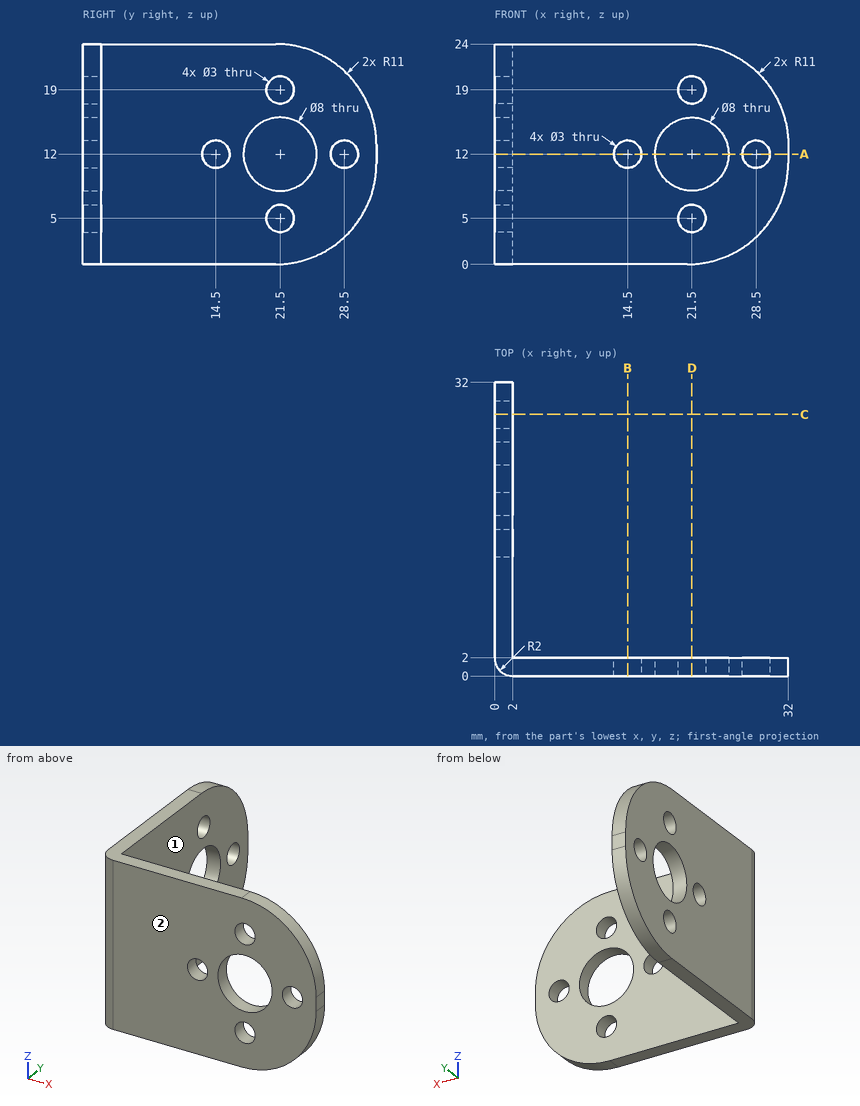
Check sheet for the drawn part. Datum: minimum x, y, z corner. Units: mm. A direction names the side the tool comes from. Round coordinates to 2 decimals unless told otherwise and drop trailing zeros. Order: outer loops, then holes, each group sorted by start corner. A loop starts at its lowest first (then second) coordinate and runs counter-clockwise, first axis right, second up. Notation, with made-up numbers: (56.5, -22.75) -> (79.5, -22.75) arc R23 cw to (79.5, -9.75) -> close; hole circle Ø2 at (-25, 78). An arc over 180 degrees is marked (long way). Put each result on its own line as item: value. Start each with the question number.
(1) Section check A-A (z = 12). State how many separate pieces and enclosed holes the cut face has, then the cut area to 3 significant figures.
(2) Section check B-B (x = 14.5). Enter the section's corners in (y, z), then the cut area to 3 significant figures.
(3) Material ranges on line 1 along Z through (x, y) = (0.65, 14.5); line 2 along X through (y, z) = (0.75, 12); line 3 along Z through (x, y) = (1, 21), recorded low to high.
(4) Depth check by flat-ended pin: pin 1 Ø1.8 at (x, z) = (21.5, 19) entering from -Y; pin 2 Ø4 at (x, z) = (21.5, 5) entering from +Y. Enter the tip coordinate at first touch or a pass-through.
(5) Section check D-D (x = 21.5). Enter the section's corners in (y, z).
(6) Section check C-C (y = 28.5). Enter the section's corners in (x, z).
(7) Tool access check on the marked faces 1 and 2. Record the directions out of +Z, -Z, +X, -X, +Y, -Y that give a thin tool (end or side, any length) a straight path to the whole face; none if there is none.
Completed:
1. separate pieces: 7
1. enclosed holes: 0
1. area: 67.1 mm2
2. outline: (0, 0) -> (2, 0) -> (2, 10.5) -> (0, 10.5) -> close; (0, 13.5) -> (2, 13.5) -> (2, 24) -> (0, 24) -> close
2. area: 42.0 mm2
3. line 1: z = 0 to 10.5, 13.5 to 24
3. line 2: x = 0.44 to 13, 16 to 17.5, 25.5 to 27, 30 to 32
3. line 3: z = 0 to 3.59, 6.41 to 8.03, 15.97 to 17.59, 20.41 to 24
4. pin 1: passes through
4. pin 2: stops at y = 2
5. outline: (0, 0.01) -> (2, 0.01) -> (2, 3.5) -> (0, 3.5) -> close; (0, 6.5) -> (2, 6.5) -> (2, 8) -> (0, 8) -> close; (0, 16) -> (2, 16) -> (2, 17.5) -> (0, 17.5) -> close; (0, 20.5) -> (2, 20.5) -> (2, 23.99) -> (0, 23.99) -> close
6. outline: (0, 2.95) -> (2, 2.95) -> (2, 10.5) -> (0, 10.5) -> close; (0, 13.5) -> (2, 13.5) -> (2, 21.05) -> (0, 21.05) -> close
7. face 1: +Z, -Z, +X, +Y
7. face 2: +Z, -Z, +X, -X, -Y
